Geometry: final body of the model. Coordinates: model frame, mm. Give positions to 0.01 mm unless a question says otherwise; leave off trailing zeros. Loops run counter-clockwise (first coordinate to the right, second up) from the corner with the lowest first, then second, coordinate; pieces in that order, holes last.
1. Material intervals for line 1 along Z through (x, y) = (2.25, 1.5); line 2 along X through (y, z) = (2, -33.5); line 3 along Z through (x, y) = (-0.25, 4), sorted ascending.
2. Section A-A, the plane z = 2. Output: boundary loops of the cut face in (x, y).
3. First-contact query: P1, Ø3, axis at x = -1.5, z = -17, coming from the +Y side; P2, Ø3, axis at y = 2.5, z = 25.5, coming from the +X side. Flat tips, straight axial feed; report the tip coordinate or a pass-through.
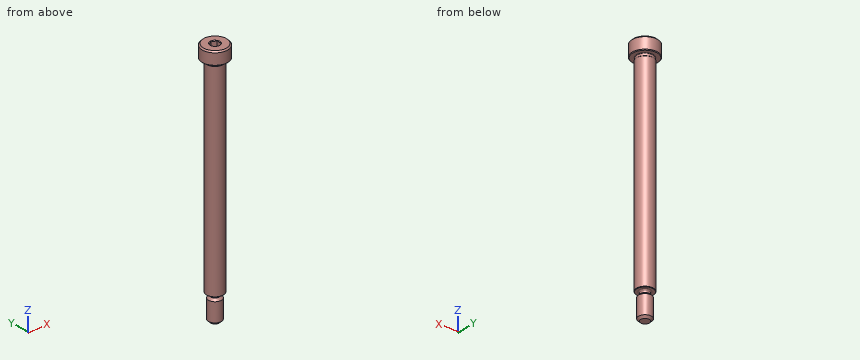
from build123d import *

# Parameters (mm, degrees)
CUT_EXTRUDE1_DEPTH = 3.095625
SKETCH5_R          = 1.833087105
CUT_EXTRUDE2_DEPTH = 3.095625
CUT_EXTRUDE2_DRAFT = -45


with BuildPart() as part:
    # Sketch3 → Revolve1 (revolve)
    with BuildSketch(Plane(origin=(0, 0, 0), x_dir=(0, 0, -1), z_dir=(1, 0, 0))):
        with BuildLine():
            Line((-45.24375, 0), (-45.24375, 4.28625))
            Line((-45.24375, 4.28625), (-44.7675, 4.7625))
            Line((-44.7675, 4.7625), (-40.719375, 4.7625))
            Line((-40.719375, 4.7625), (-40.48125, 4.524375))
            Line((-40.48125, 4.524375), (-40.48125, 3.09768875))
            ThreePointArc((-40.48125, 3.09768875), (-40.446795872, 3.014509128), (-40.36361625, 2.980055))
            Line((-40.36361625, 2.980055), (-39.579761667, 2.980055))
            Line((-39.579761667, 2.980055), (-39.422916667, 3.1369))
            Line((-39.422916667, 3.1369), (35.561905, 3.1369))
            Line((35.561905, 3.1369), (35.71875, 2.980055))
            Line((35.71875, 2.980055), (35.71875, 2.016125))
            ThreePointArc((35.71875, 2.016125), (35.834991996, 1.735491996), (36.115625, 1.61925))
            Line((36.115625, 1.61925), (36.777083333, 1.61925))
            Line((36.777083333, 1.61925), (37.570833333, 2.413))
            Line((37.570833333, 2.413), (44.45, 2.413))
            Line((44.45, 2.413), (45.24375, 1.61925))
            Line((45.24375, 1.61925), (45.24375, 0))
            Line((45.24375, 0), (-45.24375, 0))
        make_face()
    revolve(axis=Axis((0, 0, 45.24375), (0, 0, -1)))

    # Sketch4 → Cut-Extrude1 (cut)
    with BuildSketch(Plane.XY.offset(45.24375)):
        Polygon((-1.5875, -0.916543552), (0, -1.833087105), (1.5875, -0.916543552), (1.5875, 0.916543552), (0, 1.833087105), (-1.5875, 0.916543552), align=None)
    extrude(amount=-CUT_EXTRUDE1_DEPTH, mode=Mode.SUBTRACT)


with BuildPart() as cut_extrude2_tool:
    # Sketch5 → Cut-Extrude2 (with draft: the straight prism first)
    with BuildSketch(Plane.XY.offset(45.24375)):
        Circle(SKETCH5_R)
    extrude(amount=-CUT_EXTRUDE2_DEPTH)
    # Cut-Extrude2: the draft: its side faces are tilted about the plane it starts from
    cut_extrude2_sides = [cut_extrude2_tool.faces().sort_by_distance(p)[0] for p in [
        (-1.833087105, 0, 43.6959375),
    ]]
    draft(cut_extrude2_sides, Plane.XY.offset(45.24375), CUT_EXTRUDE2_DRAFT)


with BuildPart() as part_1:
    add(part.part)

    # Cut-Extrude2: cut by cut_extrude2_tool
    add(cut_extrude2_tool.part, mode=Mode.SUBTRACT)


solid = part_1.part
Answers below:
1. line 1: z = -35.72 to 45.24
1. line 2: x = -2.42 to 2.42
1. line 3: z = 40.48 to 45.24
2. outline: circle Ø6.27 at (0, 0)
3. P1: stops at y = 3.14
3. P2: stops at x = 2.97
